The model under review builds one solid part; all positions refer to its coordinate system, in mm. A direction names the side the tool comes from. Coordinates: 2 decimals unless noted, no trailing zeros. Loops run counter-clockwise (first coordinate to the right, second up) from the corner with the lowest first, then second, coordinate; pieces in that order, holes last. Notation, with made-up numbers: M 53.5,37 L 87.5,37 A23 ccw 87.5,65 Z; hole C 60,-38 d3. An arc over 180 degrees is marked long. Write item = value, one per line. Start each with the question number.
Q1. For faces 4 (the face through (-181.24, 34.96, 0.99)), 5 (the face through (-163.16, -60.23, 0.99)), 6 (the face through (-170, -17, 0)), list the 3-axis set-ups (+Z, -Z, +X, -X, +Y, -Y) from which the entire face can be reached by the end or side of a thin tool; tool diameter is ignored.
Q2. Mouldability with a two-part tool opening along Y and no side actions: class faces 1 (the face through (-158.177, 40.675, 0.986)), 2 (the face through (-157.992, -1.394, 0.986)), 3 (the face through (-160.07, -87.6, 0.99)) as released by +Y, released by -Y, zero draft, split by the parting line, or undercut.
Q3. We need section B-B on x = -174.5. Count the separate pieces of the cut face and the enclosed holes in it, and give its area (3 significant figures).
Q4. We need section A-A on x = -212. Give the boundary of the cut face in (y, z), and give its area (3 significant figures).
Q5. Wall thickness on probe 1 along Y at (x, z) = (-167, 0.5); probe 2 along Y at (x, z) = (-154.5, 1.4); probe 3 along Y at (x, z) = (-129.5, 1.05): over which ranges is each line inside the solid? List them lowest first.
Q6. We need section C-C on y = 19.5. Give the boundary of the cut face in (x, z).
Q7. We need section D-D on y = 40. Give the boundary of the cut face in (x, z).
from build123d import *

# Parameters (mm, degrees)
F1_DEPTH = 2


with BuildPart() as f1:
    # F0 (on Top) → F1 (new body)
    with BuildSketch(Plane.XY):
        with BuildLine():
            add(Edge.make_bspline(
                [(-91.6036099134, 5.71869458), (-154.910440363, -9.9027774504), (-262.0281262764, -54.2071160334), (-157.9037835768, -50.2629770203), (-91.6036099134, -47.1001818306)],
                knots=[0.3313622072, 0.3313622072, 0.3313622072, 0.3313622072, 0.5006095241, 0.683224348, 0.683224348, 0.683224348, 0.683224348], degree=3))
            Line((-91.6036099134, 5.71869458), (-226.6409774689, 76.6244625735))
            Line((-226.6409774689, 76.6244625735), (-226.6409774689, 60.3104606271))
            Line((-226.6409774689, 60.3104606271), (-134.5508992672, 8.8887251914))
            Line((-134.5508992672, 8.8887251914), (-182.0986121893, -11.9680119678))
            ThreePointArc((-182.0986121893, -11.9680119678), (-221.3284847236, -31.4249569037), (-188.3358003152, -60.2179835043))
            Line((-188.3358003152, -60.2179835043), (-182.0986121893, -57.6333925128))
            Line((-182.0986121893, -57.6333925128), (-143.684377288, -62.8968811712))
            Line((-143.684377288, -62.8968811712), (-226.6409774689, -111.9654029608))
            Line((-226.6409774689, -111.9654029608), (-226.6409774689, -126.9742846489))
            Line((-226.6409774689, -126.9742846489), (-91.6036099134, -47.1001818306))
        make_face()
    extrude(amount=F1_DEPTH)


solid = f1.part
Returned:
q1.face_4 = +Z, -Z, -X
q1.face_5 = +Z, -Z
q1.face_6 = -Z, +X, -X, +Y, -Y
q2.face_1 = released by +Y
q2.face_2 = undercut
q2.face_3 = released by -Y
q3.separate_pieces = 4
q3.enclosed_holes = 0
q3.area = 108 mm^2
q4.outline = M -118.31,0 L -103.31,0 L -103.31,2 L -118.31,2 Z; M -55.09,0 L -14.51,0 L -14.51,2 L -55.09,2 Z; M 52.14,0 L 68.94,0 L 68.94,2 L 52.14,2 Z
q4.area = 145 mm^2
q5.probe_1 = -91.7 to -76.69, -59.7 to -49.62, -17.47 to -5.35, 27.01 to 45.31
q5.probe_2 = -84.3 to -69.29, -61.41 to -49.5, -12.87 to 0.14, 20.03 to 38.74
q5.probe_3 = -69.52 to -48.77, -4.69 to 25.62
q6.outline = M -153.55,0 L -117.85,0 L -117.85,2 L -153.55,2 Z
q7.outline = M -190.27,0 L -156.89,0 L -156.89,2 L -190.27,2 Z
